from build123d import *

# Parameters (mm, degrees)
SKETCH1_W           = 100
SKETCH1_H           = 60
BOSS_EXTRUDE1_DEPTH = 50
SKETCH2_W           = 95
SKETCH2_H           = 40
CUT_EXTRUDE1_DEPTH  = 55
SKETCH3_R           = 7.5
CUT_EXTRUDE2_DEPTH  = 101


with BuildPart() as part:
    # Sketch1 → Boss-Extrude1 (new body)
    with BuildSketch(Plane.XY):
        with Locations((50, 30)):
            Rectangle(SKETCH1_W, SKETCH1_H)
    extrude(amount=BOSS_EXTRUDE1_DEPTH)

    # Sketch2 → Cut-Extrude1 (cut)
    with BuildSketch(Plane.XZ):
        with Locations((50, 25)):
            Rectangle(SKETCH2_W, SKETCH2_H)
    extrude(amount=-CUT_EXTRUDE1_DEPTH, mode=Mode.SUBTRACT)

    # Sketch3 → Cut-Extrude2 (cut, through all)
    with BuildSketch(Plane.ZY):
        with Locations((25, 20)):
            Circle(SKETCH3_R)
    extrude(amount=-CUT_EXTRUDE2_DEPTH, mode=Mode.SUBTRACT)


solid = part.part
Check sheet for the modelled part. Datum: model origin and axes. Units: mm. A direction names the side the tool comes from. Give positions to 0.01 mm unless a question says otherwise; leave off trailing zeros. Order: outer loops, then holes, each group sorted by start corner. A loop starts at its lowest first (then second) coordinate and runs counter-clockwise, first axis right, second up. Notation, with made-up numbers: (20, 62) - (43, 62) arc R29 ccw to (43, 90) - close; hole circle Ø7 at (-31.75, 24.5). An arc over 180 degrees is marked (long way). Answer as CSV lines item,"result".
1. Scan lines: probe 1 along X at (y, z) = (37, 36); probe 2 along Z at (x, y) = (81.5, 30); probe 3 along Y at (x, z) = (0.9, 25). Record each from-to range of solid material in increasing order. Write a range as from..to.
Result sheet:
probe 1,"0..2.5, 97.5..100"
probe 2,"0..5, 45..50"
probe 3,"0..12.5, 27.5..60"
2. Section check B-B (y = 20). Record the boundary of the cut face in (x, z), then the cut area to 4 significant figures.
Result sheet:
outline,"(0, 0) - (100, 0) - (100, 17.5) - (97.5, 17.5) - (97.5, 5) - (2.5, 5) - (2.5, 17.5) - (0, 17.5) - close; (0, 32.5) - (2.5, 32.5) - (2.5, 45) - (97.5, 45) - (97.5, 32.5) - (100, 32.5) - (100, 50) - (0, 50) - close"
area,"1,125 mm²"
3. Section check A-A (z = 25). Record the boundary of the cut face in (x, y).
Result sheet:
outline,"(0, 0) - (2.5, 0) - (2.5, 12.5) - (0, 12.5) - close; (0, 27.5) - (2.5, 27.5) - (2.5, 55) - (97.5, 55) - (97.5, 27.5) - (100, 27.5) - (100, 60) - (0, 60) - close; (97.5, 0) - (100, 0) - (100, 12.5) - (97.5, 12.5) - close"
4. Section check C-C (x = 76). Record the boundary of the cut face in (y, z), then the cut area to 3 significant figures.
Result sheet:
outline,"(0, 0) - (60, 0) - (60, 50) - (0, 50) - (0, 45) - (55, 45) - (55, 5) - (0, 5) - close"
area,"800 mm²"
5. Tool access check on faces 1 (the face through (100, 30, 25)), 2 (the face through (49, 27, 5)). Record the directions out of +Z, -Z, +X, -X, +Y, -Y that give a thin tool (end or side, any length) a straight path to the whole face; none if there is none.
Result sheet:
face 1,"+Z, -Z, +X, +Y, -Y"
face 2,"-Y"
6. Mould release check, pull along X, two halves, no side actions. Record for faces 3 (the face through (49, 55, 25)), 4 (the face through (46.1, 0, 45.3)), 5 (the face through (0, 30, 25)), 6 (the face through (49, 27, 45)): released by +X, released by -X, zero draft, split by the parting line, or undercut.
Result sheet:
face 3,"undercut"
face 4,"zero draft"
face 5,"released by -X"
face 6,"undercut"
7. Go/stop test with a flat-tipped pin: P1, Ø20, axis at x = 53, z = 23.5, coming from the -Y side. Record where the tip stops, or that it passes through.
Result sheet:
P1,"y = 55"
8. Section check D-D (z = 37). Record the boundary of the cut face in (x, y), then the cut area to 3 significant figures.
Result sheet:
outline,"(0, 0) - (2.5, 0) - (2.5, 55) - (97.5, 55) - (97.5, 0) - (100, 0) - (100, 60) - (0, 60) - close"
area,"775 mm²"
